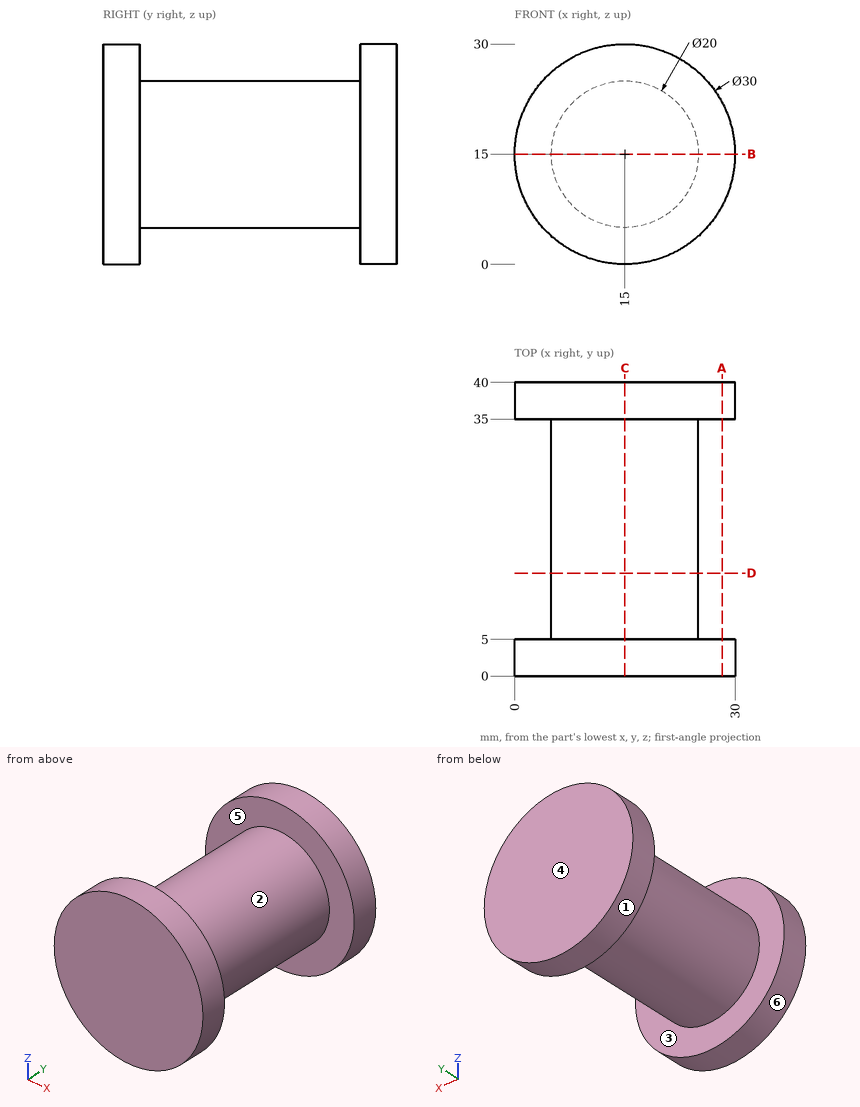
Could you check a few things on this drawing? It's one solid part, dimensions in mm from its lowest x, y, z. A direction names the side the tool comes from. Round coordinates to 2 decimals unless told otherwise and drop trailing zeros. Write each loop counter-clockwise with the first axis right and the second up, starting at its lowest first coordinate (ties: lowest second). Pieces come first, ordered by that corner, then holes. Notation, with made-up numbers: (52.25, 81) -> (61.25, 81) arc R16 ccw to (61.25, 107) -> close; hole circle Ø2 at (10.5, 67). An arc over 180 degrees is marked (long way). One line per question, with ' | ' between items. Start each with the question number.
1) On a 3-axis mill with a long thin cutter (end or side, diameter ignored), from which of +Z, -Z, +X, -X, +Y, -Y can I reach the whole of each face in a straight line? I mean the marked faces 5 and 6. Say none if no direction works.
2) Suppose I cut it at B-B on z = 15. Write out the boundary of the cut face in (x, y), then the cut area to 3 significant figures.
3) I'm going to push flat-ended pins straight in: P1, Ø12, axis at y = 17, z = 12, coming from the -X side; P2, Ø1, axis at y = 16, z = 22, coming from the -X side; P3, Ø2, axis at y = 32.5, z = 25, coming from the +X side. Where does each tip first touch, or does it pass through?
4) I need wall thicknesses on line 1 (Y direction, x = 8.75, z = 24.75); line 2 (Z direction, x = 19.5, y = 24); line 3 (X direction, y = 21.5, z = 6.75). Which ranges of each line are inside material? Lowest first, please. Write a range as [from, to].
5) If we mould it in two halves opening along Y, with no side actions, what happens to the marked faces 1, 2, 3 and 4? For each: released by +Y, released by -Y, zero draft, split by the parting line, or undercut.
6) Suppose I cut it at A-A on x = 28.25. Write out the boundary of the cut face in (y, z), then the cut area to 3 significant figures.
7) Suppose I cut it at C-C on x = 15. Write out the boundary of the cut face in (y, z), then the cut area to 3 significant figures.
8) Suppose I cut it at D-D on y = 14. Write out the boundary of the cut face in (x, z), then the cut area to 3 significant figures.
Return value:
1) face 5: none | face 6: +Y, -Y
2) outline: (0, 0) -> (30, 0) -> (30, 5) -> (25, 5) -> (25, 35) -> (30, 35) -> (30, 40) -> (0, 40) -> (0, 35) -> (5, 35) -> (5, 5) -> (0, 5) -> close | area: 900 mm2
3) P1: stops at x = 5 | P2: stops at x = 7.4 | P3: stops at x = 19.36
4) line 1: y = [0, 5], [35, 40] | line 2: z = [6.07, 23.93] | line 3: x = [9.35, 20.65]
5) face 1: zero draft | face 2: undercut | face 3: undercut | face 4: released by +Y
6) outline: (0, 7.97) -> (5, 7.97) -> (5, 22.03) -> (0, 22.03) -> close; (35, 7.97) -> (40, 7.97) -> (40, 22.03) -> (35, 22.03) -> close | area: 141 mm2
7) outline: (0, 0) -> (5, 0) -> (5, 5) -> (35, 5) -> (35, 0) -> (40, 0) -> (40, 30) -> (35, 30) -> (35, 25) -> (5, 25) -> (5, 30) -> (0, 30) -> close | area: 900 mm2
8) outline: circle Ø20 at (15, 15) | area: 314 mm2
